Autodesk Inventor part; units mm, degrees
ref_plane "Work Plane3" through (6.6548, -916.4402, 6.985) normal (0, 0, -1) x (0, 1, 0)
ref_plane "YZ Plane" through (0, 0, 0) normal (1, 0, 0) x (0, 1, 0)
ref_plane "XZ Plane" through (0, 0, 0) normal (0, 1, 0) x (-1, 0, 0)
ref_plane "Work Plane1" through (0, 0, 0) normal (0, 0, 1) x (1, 0, 0)
ref_plane "Work Plane2" through (0, 0, 0) normal (0, 0, 1) x (1, 0, 0)
sketch "Sketch2" plane through (0, 0, 0) normal (0, 0, 1) x (1, 0, 0)
  line L0 (1.9142, -654.4) -> (1.9142, -1000) construction
  line L1 (13.0858, -1000) -> (13.0858, -654.4) construction
  line L2 (10.8204, -900) -> (1.905, -900) construction
  line L3 (1.1684, -919.8882) -> (10.8204, -919.8882) construction
  circle A0 centre (8.3884, -914.7066) radius 1.1938 construction
  circle A1 centre (8.3884, -905.1816) radius 1.1938 construction
  line L4 (1.9142, -930.0482) -> (13.0858, -930.0482)
  line L5 (13.0858, -930.0482) -> (13.0858, -889.84)
  line L6 (13.0858, -889.84) -> (1.9142, -889.84)
  line L7 (1.9142, -889.84) -> (1.9142, -930.0482)
  circle A2 centre (7.5, -924.8932) radius 1.7
  circle A3 centre (7.5, -894.995) radius 1.7
  circle A4 centre (5.8484, -914.7066) radius 1.4097 construction
  circle A5 centre (5.8484, -914.7066) radius 3.4925 construction
  circle A6 centre (10.9284, -914.7066) radius 1.4097 construction
  circle A7 centre (10.9284, -914.7066) radius 3.4925 construction
  line L8 (5.8484, -914.7066) -> (10.9284, -914.7066) construction
  line L9 (5.8484, -916.1163) -> (10.9284, -916.1163)
  line L10 (10.9284, -913.2969) -> (5.8484, -913.2969)
  arc A8 (5.8484, -913.2969) -> (5.8484, -916.1163) centre (5.8484, -914.7066) ccw
  arc A9 (10.9284, -916.1163) -> (10.9284, -913.2969) centre (10.9284, -914.7066) ccw
  circle A10 centre (10.9284, -905.1816) radius 1.4097 construction
  circle A11 centre (10.9284, -905.1816) radius 3.4925 construction
  line L11 (5.8484, -906.5913) -> (10.9284, -906.5913)
  line L12 (10.9284, -903.7719) -> (5.8484, -903.7719)
  arc A12 (5.8484, -903.7719) -> (5.8484, -906.5913) centre (5.8484, -905.1816) ccw
  arc A13 (10.9284, -906.5913) -> (10.9284, -903.7719) centre (10.9284, -905.1816) ccw
  point P0 (0, 0)
  dimension "d0" = 10.16
  dimension "d1" = 10.16
  dimension "d4" = 3.4
  dimension "d5" = 3.4
  dimension "d6" = 5.155
  dimension "d7" = 5.155
  dimension "d8" = 2.8194
  dimension "d9" = 2.54
  dimension "d10" = 6.985
  dimension "d11" = 2.8194
  dimension "d12" = 6.985
  dimension "d13" = 2.54
  dimension "d14" = 2.8194
  dimension "d15" = 2.8194
  dimension "d16" = 6.985
  dimension "d17" = 2.8194
ref_plane "Work Plane3" through (6.6548, -916.4402, 6.985) normal (0, 0, -1) x (0, 1, 0)
extrude "Extrusion1" add sketch "Sketch2" along normal up to surface (6.985 mm away)
sketch "Sketch3" plane through (0, 0, 0) normal (0, 0, -1) x (-1, 0, 0)
  arc A0 (-5.8484, -906.5913) -> (-5.8484, -903.7719) centre (-5.8484, -905.1816) ccw construction
  arc A1 (-10.9284, -903.7719) -> (-10.9284, -906.5913) centre (-10.9284, -905.1816) ccw construction
  line L0 (-5.8484, -905.1816) -> (-10.9284, -905.1816) construction
  line L1 (-10.9284, -906.5913) -> (-5.8484, -906.5913) construction
  line L2 (-8.3884, -906.5913) -> (-8.3884, -903.7719) construction
  line L3 (-5.8484, -913.2969) -> (-10.9284, -913.2969) construction
  line L4 (-8.3884, -913.2969) -> (-8.3884, -916.1163) construction
  line L5 (-10.9284, -916.1163) -> (-5.8484, -916.1163) construction
  arc A2 (-5.8484, -916.1163) -> (-5.8484, -913.2969) centre (-5.8484, -914.7066) ccw construction
  arc A3 (-10.9284, -913.2969) -> (-10.9284, -916.1163) centre (-10.9284, -914.7066) ccw construction
  line L6 (-5.8484, -914.7066) -> (-10.9284, -914.7066) construction
  line L7 (-13.0858, -930.0482) -> (-13.0858, -889.84)
  line L8 (-1.9142, -908.6741) -> (-13.0858, -908.6741)
  line L9 (-13.0858, -908.6741) -> (-13.0858, -901.6891)
  line L10 (-13.0858, -901.6891) -> (-1.9142, -901.6891)
  line L11 (-3.6909, -908.6741) -> (-13.0858, -901.6891) construction
  line L12 (-13.0858, -908.6741) -> (-3.6909, -901.6891) construction
  line L13 (-1.9142, -889.84) -> (-1.9142, -930.0482) construction
  line L14 (-1.9142, -901.6891) -> (-1.9142, -908.6741)
  line L15 (-1.9142, -889.84) -> (-1.9142, -930.0482)
  line L16 (-1.9142, -918.1991) -> (-13.0858, -918.1991)
  line L17 (-13.0858, -918.1991) -> (-13.0858, -911.2141)
  line L18 (-13.0858, -911.2141) -> (-1.9142, -911.2141)
  line L19 (-1.9142, -911.2141) -> (-1.9142, -918.1991)
  point P0 (0, 0)
  point P1 (-8.3884, -905.1816)
  dimension "d20" = 6.985
  dimension "d21" = 6.985
extrude "Nut Well" cut sketch "Sketch3" against normal blind 4.572 contours L7 L18 L15 L16 | L7 L10 L14 L8
fillet "Fillet1" radius 3.175 4 edges at (13.0858, -889.84, 3.4925) (13.0858, -930.0482, 3.4925) (1.9142, -930.0482, 3.4925) (1.9142, -889.84, 3.4925)
equation "\"d1\" = d0"
equation "\"d7\" = d6"
properties part number "Limit swtich mount bottom"
CAD build for the part. Positions are in the model's coordinates, mm. A direction names the side the tool comes from. Give positions to 0.01 mm unless a question says otherwise; leave off trailing zeros. Write each loop counter-clockwise with the first axis right and the second up, starting at its lowest first coordinate (ties: lowest second). Pieces come first, ordered by that corner, then holes. Notation, with made-up numbers: M 31.5,-21.5 L 67.5,-21.5 A27 cw 67.5,-0.5 Z; hole C -13.75,84 d2. An arc over 180 degrees is marked long. Return JSON: item names as keys, results as strings. Group by question number.
(1) 3-axis set-ups, long thin cutter, end or side, ignore diameter. For faces 4 (the face through (1.914, -910, 4)), 5 (the face through (7, -918.199, 2)), 6 (the face through (12.338, -914.676, 5.762)): which of +Z, -Z, +X, -X, +Y, -Y reach the whole face in a straight line?
(2) Band-saw the part on D-D (y = -917). Give the cut face in (x, z) (3 decimals).
(3) Drill centre lines: L1, parallel to Y at x = 7.5, z = 2.75 (3 decimals); L2, parallel to Y at x = 10, z = 5; L3, parallel to Y at x = 9.5, z = 1.5. Where is each one in solid material? Low to high. Write a range as [from, to].
(4) Flat gauge pins, fed straight in: pin 1 Ø2.5 at (x, y) = (7.5, -924.89) entering from -Z; pin 2 Ø3 at (x, z) = (3, 2.5) entering from -Y. Where does each tip first touch, or does it go through?
(5) Band-saw the part on C-C (x = 11.5). Give the cut face in (y, z) (3 decimals).
(6) Mould opens along X. For faces 1 (the face through (12.18, -890.795, 3.541)), 2 (the face through (8, -911.214, 2)), 3 (the face through (8, -906.591, 6)) say: pulls with the +X half, pulls with the -X half, needs draft (parallel to the pull), parting line crosses it, or undercut.
(7) Band-saw the part on A-A (x = 7.5). Give the cut face in (y, z) (3 decimals).
(8) Band-saw the part on B-B (z = 2.25). Give the cut face in (x, y) (3 decimals), and give its area (3 significant figures).
Entries:
{
 "1": {"face 4": "+Z, -Z, -X, +Y, -Y", "face 5": "-Z, +X, -X", "face 6": "+Z, -Z"},
 "2": {"outline": "M 1.914,4.572 L 13.086,4.572 L 13.086,6.985 L 1.914,6.985 Z"},
 "3": {"L1": "y = [-930.048, -926.593], [-923.193, -918.199], [-911.214, -908.674], [-901.689, -896.695], [-893.295, -889.84]", "L2": "y = [-930.05, -916.12], [-913.3, -906.59], [-903.77, -889.84]", "L3": "y = [-930.05, -918.2], [-911.21, -908.67], [-901.69, -889.84]"},
 "4": {"pin 1": "passes through", "pin 2": "stops at y = -929.99"},
 "5": {"outline": "M -929.622,0 L -918.199,0 L -918.199,4.572 L -915.995,4.572 L -915.995,6.985 L -929.622,6.985 Z; M -913.418,4.572 L -911.214,4.572 L -911.214,0 L -908.674,0 L -908.674,4.572 L -906.47,4.572 L -906.47,6.985 L -913.418,6.985 Z; M -903.893,4.572 L -901.689,4.572 L -901.689,0 L -890.266,0 L -890.266,6.985 L -903.893,6.985 Z"},
 "6": {"face 1": "pulls with the +X half", "face 2": "needs draft", "face 3": "undercut"},
 "7": {"outline": "M -930.048,0 L -926.593,0 L -926.593,6.985 L -930.048,6.985 Z; M -923.193,0 L -918.199,0 L -918.199,4.572 L -916.116,4.572 L -916.116,6.985 L -923.193,6.985 Z; M -913.297,4.572 L -911.214,4.572 L -911.214,0 L -908.674,0 L -908.674,4.572 L -906.591,4.572 L -906.591,6.985 L -913.297,6.985 Z; M -903.772,4.572 L -901.689,4.572 L -901.689,0 L -896.695,0 L -896.695,6.985 L -903.772,6.985 Z; M -893.295,0 L -889.84,0 L -889.84,6.985 L -893.295,6.985 Z"},
 "8": {"outline": "M 1.914,-926.873 A3.175 ccw 5.089,-930.048 L 9.911,-930.048 A3.175 ccw 13.086,-926.873 L 13.086,-918.199 L 1.914,-918.199 Z; M 1.914,-911.214 L 13.086,-911.214 L 13.086,-908.674 L 1.914,-908.674 Z; M 1.914,-901.689 L 13.086,-901.689 L 13.086,-893.015 A3.175 ccw 9.911,-889.84 L 5.089,-889.84 A3.175 ccw 1.914,-893.015 Z; hole C 7.5,-924.893 d3.4; hole C 7.5,-894.995 d3.4", "area": "266 mm^2"}
}
